Part model, mm, in its own coordinate system. A direction names the side the tool comes from. Give positions to 0.01 mm unless a question says otherwise; leave off trailing zeros. Order: outer loops, then holes, each group sorted by start corner. A loop starts at its lowest first (then second) coordinate and runs counter-clockwise, first axis right, second up. Notation, with made-up numbers: (-37, 8) - (-31, 8) arc R36 cw to (-31, 45) - close; hole circle Ø9 at (82.5, -7.5). An arc over 180 degrees is marked (long way). One line per item, written item: value.
```python
from build123d import *

# Parameters (mm, degrees)
SKETCH1_W           = 70
SKETCH1_H           = 130
BOSS_EXTRUDE1_DEPTH = 4
CUT_EXTRUDE1_DEPTH  = 148.702403501
SKETCH3_W           = 23
SKETCH3_H           = 6
SKETCH3_W_2         = 6
SKETCH3_H_2         = 26
CUT_EXTRUDE2_DEPTH  = 148.702403501


with BuildPart() as part:
    # Sketch1 → Boss-Extrude1 (new body)
    with BuildSketch(Plane(origin=(0, 0, 0), x_dir=(1, 0, 0), z_dir=(0, 1, 0))):
        with Locations((35, 65)):
            Rectangle(SKETCH1_W, SKETCH1_H)
    extrude(amount=BOSS_EXTRUDE1_DEPTH)

    # Sketch2 → Cut-Extrude1 (cut, through all)
    with BuildSketch(Plane(origin=(0, 4, 0), x_dir=(1, 0, 0), z_dir=(0, 1, 0))):
        with BuildLine():
            ThreePointArc((17, 79.5), (12.732233047, 81.267766953), (14.5, 77))
            Line((14.5, 77), (14.5, 79.5))
            Line((14.5, 79.5), (17, 79.5))
        make_face()
        with BuildLine():
            Line((14.5, 79.5), (14.5, 77))
            ThreePointArc((14.5, 77), (16.267766953, 77.732233047), (17, 79.5))
            Line((17, 79.5), (14.5, 79.5))
        make_face()
        with BuildLine():
            Line((14.5, 53), (14.5, 50.5))
            Line((14.5, 50.5), (17, 50.5))
            ThreePointArc((17, 50.5), (16.267766953, 52.267766953), (14.5, 53))
        make_face()
        with BuildLine():
            Line((17, 50.5), (14.5, 50.5))
            Line((14.5, 50.5), (14.5, 53))
            ThreePointArc((14.5, 53), (12.732233047, 48.732233047), (17, 50.5))
        make_face()
        with BuildLine():
            ThreePointArc((43.5, 53), (41.732233047, 52.267766953), (41, 50.5))
            Line((41, 50.5), (43.5, 50.5))
            Line((43.5, 50.5), (43.5, 53))
        make_face()
        with BuildLine():
            Line((43.5, 50.5), (41, 50.5))
            ThreePointArc((41, 50.5), (43.5, 48), (46, 50.5))
            ThreePointArc((46, 50.5), (45.267766953, 52.267766953), (43.5, 53))
            Line((43.5, 53), (43.5, 50.5))
        make_face()
        with BuildLine():
            ThreePointArc((41, 79.5), (41.732233047, 77.732233047), (43.5, 77))
            Line((43.5, 77), (43.5, 79.5))
            Line((43.5, 79.5), (41, 79.5))
        make_face()
        with BuildLine():
            Line((43.5, 79.5), (43.5, 77))
            ThreePointArc((43.5, 77), (45.267766953, 77.732233047), (46, 79.5))
            ThreePointArc((46, 79.5), (43.5, 82), (41, 79.5))
            Line((41, 79.5), (43.5, 79.5))
        make_face()
    extrude(amount=-CUT_EXTRUDE1_DEPTH, mode=Mode.SUBTRACT)

    # Sketch3 → Cut-Extrude2 (cut, through all)
    with BuildSketch(Plane(origin=(0, 4, 0), x_dir=(1, 0, 0), z_dir=(0, 1, 0))):
        with Locations((34.5, 3)):
            Rectangle(SKETCH3_W, SKETCH3_H)
        with Locations((67, 39)):
            Rectangle(SKETCH3_W_2, SKETCH3_H_2)
        with Locations((67, 91)):
            Rectangle(SKETCH3_W_2, SKETCH3_H_2)
        with Locations((34.5, 127)):
            Rectangle(SKETCH3_W, SKETCH3_H)
    extrude(amount=-CUT_EXTRUDE2_DEPTH, mode=Mode.SUBTRACT)


solid = part.part
```
1) Cut at A-A, the plane y = 2.05. Give the cut face in (x, z), then the cut area to 3 significant figures.
Outcome:
outline: (0, -130) - (23, -130) - (23, -124) - (46, -124) - (46, -130) - (70, -130) - (70, -104) - (64, -104) - (64, -78) - (70, -78) - (70, -52) - (64, -52) - (64, -26) - (70, -26) - (70, 0) - (46, 0) - (46, -6) - (23, -6) - (23, 0) - (0, 0) - close; hole circle Ø5 at (14.5, -79.5); hole circle Ø5 at (14.5, -50.5); hole circle Ø5 at (43.5, -79.5); hole circle Ø5 at (43.5, -50.5)
area: 8,430 mm^2
2) Pin check, flat tip, straight feed: pin 1 (1.2 mm diameter, centred on x = 38, y = 2.5, fed in from -Z). Stop position of the tip, or through.
Outcome:
pin 1: stops at z = -124
3) Mould opens along Z. For faces 4 (the flat face through (67, 2, -104)), 5 (the flat face through (58, 2, 0)), 6 (the flat face through (34, 2, -124)) say: released by +Z, released by -Z, zero draft, split by the parting line, or undercut.
Outcome:
face 4: undercut
face 5: released by +Z
face 6: released by -Z
4) Cut at B-B, the plane z = -37. Give the cut face in (x, y).
Outcome:
outline: (0, 0) - (64, 0) - (64, 4) - (0, 4) - close
5) Cut at C-C, the plane x = 33.5. Give the cut face in (y, z).
Outcome:
outline: (0, -124) - (4, -124) - (4, -6) - (0, -6) - close
6) Drill centre lines: line 1 along Z through (x, y) = (14.5, 2.9); line 2 along X through (y, z) = (2.3, -79.5); line 3 along Z through (x, y) = (14, 3.7). Where is each one in solid material? Low to high. Write a range as from..to.
Outcome:
line 1: z = -130..-82, -77..-53, -48..0
line 2: x = 0..12, 17..41, 46..64
line 3: z = -130..-81.95, -77.05..-52.95, -48.05..0
7) Which spindle directions (+Z, -Z, +X, -X, +Y, -Y) get a long thin tool onto all of the face, cutting with end or side? Do faces 1 (the flat face through (67, 2, -52)), 2 (the flat face through (23, 2, -3)), 3 (the flat face through (0, 2, -64)). Say none if no direction does.
Outcome:
face 1: +X, +Y, -Y
face 2: +Z, +Y, -Y
face 3: +Z, -Z, -X, +Y, -Y
